from build123d import *

# Parameters (mm, degrees)
F0_R     = 1.5
F1_DEPTH = 3


with BuildPart() as f1:
    # F0 (on Top) → F1 (new body)
    with BuildSketch(Plane.XY):
        with BuildLine():
            Line((15, 3), (0, 3))
            Line((0, 3), (-15, 3))
            ThreePointArc((-15, 3), (-12.87868, 2.12132), (-12, 0))
            ThreePointArc((-12, 0), (-12.87868, -2.12132), (-15, -3))
            Line((-15, -3), (0, -3))
            Line((0, -3), (15, -3))
            ThreePointArc((15, -3), (18, 0), (15, 3))
        make_face()
        with BuildLine():
            ThreePointArc((-8.5, -1.5), (-10, 0), (-8.5, 1.5))
            Line((-8.5, 1.5), (15, 1.5))
            ThreePointArc((15, 1.5), (16.06066, 1.06066), (16.5, 0))
            ThreePointArc((16.5, 0), (16.06066, -1.06066), (15, -1.5))
            Line((15, -1.5), (-8.5, -1.5))
        make_face(mode=Mode.SUBTRACT)
        with BuildLine():
            ThreePointArc((-12, 0), (-12.87868, 2.12132), (-15, 3))
            ThreePointArc((-15, 3), (-18, 0), (-15, -3))
            ThreePointArc((-15, -3), (-12.87868, -2.12132), (-12, 0))
        make_face()
        with Locations((-15, 0)):
            Circle(F0_R, mode=Mode.SUBTRACT)
    extrude(amount=F1_DEPTH)


solid = f1.part
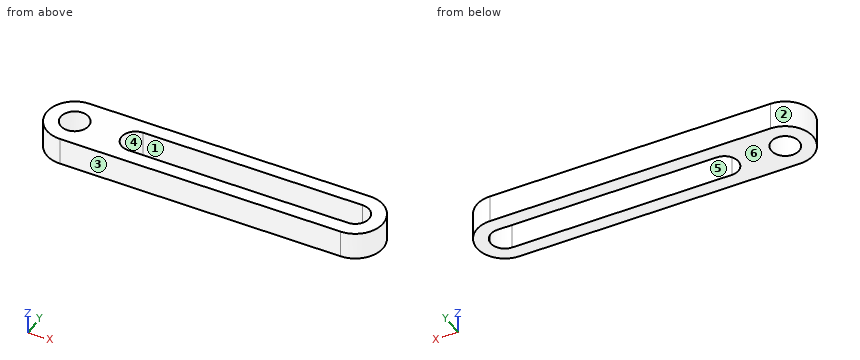
Design review of the part built by this model. Coordinates are the model's own, in mm. Face numbers are marked on the shaded views. A direction names the side the tool comes from. Coordinates: 2 decimals unless noted, no trailing zeros. Order: outer loops, then holes, each group sorted by start corner. A loop starts at its lowest first (then second) coordinate and runs counter-clockwise, first axis right, second up. Notation, with made-up numbers: (-11, -5.5) -> (9, -5.5) arc R17 ccw to (9, 18.5) -> close; hole circle Ø8 at (-30, 14). An arc over 180 degrees is marked (long way). Use one line per item in the form item = value. Start each with the question number.
(1) For probe 1 along Y at (x, z) = (1, 2.6); probe 2 along X at (y, z) = (-0.8, 0.55); probe 3 along X at (y, z) = (1.15, 1.75), list the stretches that pass through material, from the lowest coordinate up.
(2) Add section D-D on y = -0.3. State the section outline as (x, z) points.
(3) Add section C-C on z = 1.7. State the section outline as (x, y) points, plus the area to 3 significant figures.
(4) The part is to be moulded in two halves that separate along X. For the marked faces 1, 2, 3 and 4, say which applies: +X half, -X half, draft (parallel to the pull), parting line (faces both ways), or undercut.
(5) For the marked faces 5 and 6, list the 3-axis set-ups (+Z, -Z, +X, -X, +Y, -Y) from which the entire face can be reached by the end or side of a thin tool; tool diameter is ignored.
(6) Add section B-B on y = 1.1. State the section outline as (x, z) points.
(7) Add section A-A on x = -5. State the section outline as (y, z) points, plus the area to 3 significant figures.
Answer block:
q1.probe_1 = -3 to -1.5, 1.5 to 3
q1.probe_2 = -17.89 to -16.27, -13.73 to -9.77, 16.27 to 17.89
q1.probe_3 = -17.77 to -15.96, -14.04 to -9.46, 15.96 to 17.77
q2.outline = (-17.98, 0) -> (-16.47, 0) -> (-16.47, 3) -> (-17.98, 3) -> close; (-13.53, 0) -> (-9.97, 0) -> (-9.97, 3) -> (-13.53, 3) -> close; (16.47, 0) -> (17.98, 0) -> (17.98, 3) -> (16.47, 3) -> close
q3.outline = (-15, -3) -> (15, -3) arc R3 ccw to (15, 3) -> (-15, 3) arc R3 ccw to start; hole circle Ø3 at (-15, 0); hole (-8.5, -1.5) -> (15, -1.5) arc R1.5 ccw to (16.5, 0) arc R1.5 ccw to (15, 1.5) -> (-8.5, 1.5) arc R1.5 ccw to start
q3.area = 124 mm²
q4.face_1 = undercut
q4.face_2 = -X half
q4.face_3 = draft
q4.face_4 = undercut
q5.face_5 = +Z, -Z
q5.face_6 = -Z, +X, -X, +Y, -Y
q6.outline = (-17.79, 0) -> (-16.02, 0) -> (-16.02, 3) -> (-17.79, 3) -> close; (-13.98, 0) -> (-9.52, 0) -> (-9.52, 3) -> (-13.98, 3) -> close; (16.02, 0) -> (17.79, 0) -> (17.79, 3) -> (16.02, 3) -> close
q7.outline = (-3, 0) -> (-1.5, 0) -> (-1.5, 3) -> (-3, 3) -> close; (1.5, 0) -> (3, 0) -> (3, 3) -> (1.5, 3) -> close
q7.area = 9.00 mm²
